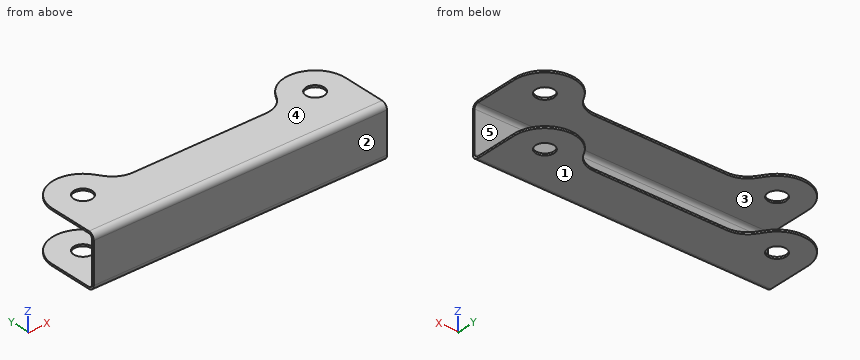
```python
from build123d import *

# Parameters (mm, degrees)
BASE_EXTRUDE_DEPTH         = 13.5
FILLET1_R                  = 12.7
SHELL1_T                   = -1
SKETCH2_R                  = 4.7625
CUT_EXTRUDE1_DEPTH         = 142.468143499
FLATTEN_BENDS1_START       = -24.4
FLATTEN_BENDS1_OUTLINE_W   = 152.4
FLATTEN_BENDS1_OUTLINE_H   = 1
FLATTEN_BENDS1_DEPTH       = 41.4
FLATTEN_BENDS1_START_2     = -25.4
FLATTEN_BENDS1_2_OUTLINE_R = 4.7625
FLATTEN_BENDS1_2_DEPTH     = 1
PROCESS_BENDS1_START       = -54
PROCESS_BENDS1_OUTLINE_W   = 152.4
PROCESS_BENDS1_OUTLINE_H   = 1
PROCESS_BENDS1_DEPTH       = 40.80822
PROCESS_BENDS1_START_2     = 13.19178
PROCESS_BENDS1_2_OUTLINE_W = 152.4
PROCESS_BENDS1_2_OUTLINE_H = 1
PROCESS_BENDS1_2_DEPTH     = 40.80822
PROCESS_BENDS1_START_3     = -13.5
PROCESS_BENDS1_3_OUTLINE_R = 4.7625
PROCESS_BENDS1_3_DEPTH     = 3
PROCESS_BENDS1_START_4     = 10.5
PROCESS_BENDS1_4_OUTLINE_R = 4.7625
PROCESS_BENDS1_4_DEPTH     = 3
PROCESS_BENDS1_START_5     = -15.875
PROCESS_BENDS1_5_DEPTH     = 152.4


with BuildPart() as part:
    # Sketch1 → Base-Extrude (new, symmetric)
    with BuildSketch(Plane.XY):
        with BuildLine():
            Line((-15.875, 0), (-15.875, -25.4))
            Line((-15.875, -25.4), (136.525, -25.4))
            Line((136.525, -25.4), (136.525, 0))
            ThreePointArc((136.525, 0), (123.40666482, 15.633823079), (105.732379645, 5.429569775))
            Line((105.732379645, 5.429569775), (103.756177862, 0))
            Line((103.756177862, 0), (19.379796597, 0))
            Line((19.379796597, 0), (13.004038703, 9.105525927))
            ThreePointArc((13.004038703, 9.105525927), (-4.773704567, 15.140256593), (-15.875, 0))
        make_face()
    extrude(amount=BASE_EXTRUDE_DEPTH, both=True)

    # Fillet1
    # the kernel refuses this fillet: 12.7 mm, written as the material it adds along each edge
    with BuildSketch(Plane(origin=(103.756177862, 0, -13.5), x_dir=(-1, 0, 0), z_dir=(0, 0, 1))) as fillet1_piece_1:
        with BuildLine():
            CenterArc((8.703846213, -12.7), FILLET1_R, 90, 63.612200039)
            Line((-2.672895276, -7.055555556), (-3.810569425, -6.491111111))
            ThreePointArc((-3.810569425, -6.491111111), (-3.169611411, -4.995204193), (-1.193409628, 0.434365582))
            Line((-1.193409628, 0.434365582), (0, 1.27))
            Line((0, 1.27), (8.703846213, 1.27))
            Line((8.703846213, 1.27), (8.703846213, 0))
        make_face()
    extrude(amount=27)
    with BuildSketch(Plane(origin=(19.379796597, 0, 13.5), x_dir=(-0.5735764363510504, 0.8191520442889888, 0), z_dir=(0, 0, -1))) as fillet1_piece_2:
        with BuildLine():
            CenterArc((FILLET1_R * 0.520567050552, FILLET1_R), FILLET1_R, 215, 55)
            Line((-FILLET1_R * 0.298584993737, FILLET1_R * 0.426423563649), (0, 0))
            Line((0, 0), (FILLET1_R * 0.520567050552, 0))
        make_face()
    extrude(amount=27)

    # Shell1
    shell1_openings = [part.faces().sort_by_distance(p)[0] for p in [
        (-15.875, -12.7, 0),
        (136.525, -12.7, 0),
        (124.273424559, 15.45595094, 0),
        (60.521664894, 0, 0),
        (14.29590294, 7.260552593, 0),
        (-4.773704567, 15.140256593, 0),
        (20.126790751, 1.434962419, 0),
        (101.745819363, 1.907075363, 0),
    ]]
    offset(amount=SHELL1_T, openings=shell1_openings, kind=Kind.INTERSECTION)

    # Sketch2 → Cut-Extrude1 (cut, through all)
    with BuildSketch(Plane.XY.offset(13.5)):
        with Locations((120.65, 0)):
            Circle(SKETCH2_R)
        Circle(SKETCH2_R)
    extrude(amount=-CUT_EXTRUDE1_DEPTH, mode=Mode.SUBTRACT)

    # Flatten-Bends1: read off the stored shape, not the designer's step
    # Flatten-Bends1 outline → Flatten-Bends1 (cut)
    with BuildSketch(Plane(origin=(0, 0, 0), x_dir=(1, 0, 0), z_dir=(0, 1, 0)).offset(FLATTEN_BENDS1_START)):
        with Locations((60.325, 13)):
            Rectangle(FLATTEN_BENDS1_OUTLINE_W, FLATTEN_BENDS1_OUTLINE_H)
        with Locations((60.325, -13)):
            Rectangle(FLATTEN_BENDS1_OUTLINE_W, FLATTEN_BENDS1_OUTLINE_H)
    extrude(amount=FLATTEN_BENDS1_DEPTH, mode=Mode.SUBTRACT)

    # Flatten-Bends1 2 outline → Flatten-Bends1 2 (add)
    # profile 1 of 2: a face of its own
    with BuildSketch(Plane(origin=(0, 0, 0), x_dir=(1, 0, 0), z_dir=(0, 1, 0)).offset(FLATTEN_BENDS1_START_2)):
        with BuildLine():
            ThreePointArc((106.429073138, -43.882546373), (124.273424559, -52.282941757), (136.525, -36.826990817))
            Line((136.525, -36.826990817), (136.525, -13.5))
            Line((136.525, -13.5), (-15.875, -13.5))
            Line((-15.875, -13.5), (-15.875, -36.826990817))
            ThreePointArc((-15.875, -36.826990817), (-4.773704567, -51.96724741), (13.004038703, -45.932516744))
            Line((13.004038703, -45.932516744), (15.587767176, -42.242570075))
            ThreePointArc((15.587767176, -42.242570075), (20.126790751, -38.261953236), (25.990998139, -36.826990817))
            Line((25.990998139, -36.826990817), (95.052331649, -36.826990817))
            ThreePointArc((95.052331649, -36.826990817), (101.745819363, -38.73406618), (106.429073138, -43.882546373))
        make_face()
        with Locations((0, -36.826990817)):
            Circle(FLATTEN_BENDS1_2_OUTLINE_R, mode=Mode.SUBTRACT)
        with Locations((120.65, -36.826990817)):
            Circle(FLATTEN_BENDS1_2_OUTLINE_R, mode=Mode.SUBTRACT)
    # profile 2 of 2: a face of its own
    with BuildSketch(Plane(origin=(0, 0, 0), x_dir=(1, 0, 0), z_dir=(0, 1, 0)).offset(FLATTEN_BENDS1_START_2)):
        with BuildLine():
            Line((-15.875, 36.826990817), (-15.875, 13.5))
            Line((-15.875, 13.5), (136.525, 13.5))
            Line((136.525, 13.5), (136.525, 36.826990817))
            ThreePointArc((136.525, 36.826990817), (124.273424559, 52.282941757), (106.429073138, 43.882546373))
            ThreePointArc((106.429073138, 43.882546373), (101.745819363, 38.73406618), (95.052331649, 36.826990817))
            Line((95.052331649, 36.826990817), (25.990998139, 36.826990817))
            ThreePointArc((25.990998139, 36.826990817), (20.126790751, 38.261953236), (15.587767176, 42.242570075))
            Line((15.587767176, 42.242570075), (13.004038703, 45.932516744))
            ThreePointArc((13.004038703, 45.932516744), (-4.773704567, 51.96724741), (-15.875, 36.826990817))
        make_face()
        with Locations((0, 36.826990817)):
            Circle(FLATTEN_BENDS1_2_OUTLINE_R, mode=Mode.SUBTRACT)
        with Locations((120.65, 36.826990817)):
            Circle(FLATTEN_BENDS1_2_OUTLINE_R, mode=Mode.SUBTRACT)
    extrude(amount=FLATTEN_BENDS1_2_DEPTH)

    # Process-Bends1: read off the stored shape, not the designer's step
    # Process-Bends1 outline → Process-Bends1 (cut)
    with BuildSketch(Plane.XY.offset(PROCESS_BENDS1_START)):
        with Locations((60.325, -24.9)):
            Rectangle(PROCESS_BENDS1_OUTLINE_W, PROCESS_BENDS1_OUTLINE_H)
    extrude(amount=PROCESS_BENDS1_DEPTH, mode=Mode.SUBTRACT)

    # Process-Bends1 2 outline → Process-Bends1 2 (cut)
    with BuildSketch(Plane.XY.offset(PROCESS_BENDS1_START_2)):
        with Locations((60.325, -24.9)):
            Rectangle(PROCESS_BENDS1_2_OUTLINE_W, PROCESS_BENDS1_2_OUTLINE_H)
    extrude(amount=PROCESS_BENDS1_2_DEPTH, mode=Mode.SUBTRACT)

    # Process-Bends1 3 outline → Process-Bends1 3 (add)
    with BuildSketch(Plane.XY.offset(PROCESS_BENDS1_START_3)):
        with BuildLine():
            Line((136.525, -24.4), (136.525, 0))
            ThreePointArc((136.525, 0), (124.273424559, 15.45595094), (106.429073138, 7.055555556))
            ThreePointArc((106.429073138, 7.055555556), (101.745819363, 1.907075363), (95.052331649, 0))
            Line((95.052331649, 0), (25.990998139, 0))
            ThreePointArc((25.990998139, 0), (20.126790751, 1.434962419), (15.587767176, 5.415579258))
            Line((15.587767176, 5.415579258), (13.004038703, 9.105525927))
            ThreePointArc((13.004038703, 9.105525927), (-4.773704567, 15.140256593), (-15.875, 0))
            Line((-15.875, 0), (-15.875, -24.4))
            Line((-15.875, -24.4), (136.525, -24.4))
        make_face()
        Circle(PROCESS_BENDS1_3_OUTLINE_R, mode=Mode.SUBTRACT)
        with Locations((120.65, 0)):
            Circle(PROCESS_BENDS1_3_OUTLINE_R, mode=Mode.SUBTRACT)
    extrude(amount=PROCESS_BENDS1_3_DEPTH)

    # Process-Bends1 4 outline → Process-Bends1 4 (add)
    with BuildSketch(Plane.XY.offset(PROCESS_BENDS1_START_4)):
        with BuildLine():
            Line((136.525, -24.4), (136.525, 0))
            ThreePointArc((136.525, 0), (124.273424559, 15.45595094), (106.429073138, 7.055555556))
            ThreePointArc((106.429073138, 7.055555556), (101.745819363, 1.907075363), (95.052331649, 0))
            Line((95.052331649, 0), (25.990998139, 0))
            ThreePointArc((25.990998139, 0), (20.126790751, 1.434962419), (15.587767176, 5.415579258))
            Line((15.587767176, 5.415579258), (13.004038703, 9.105525927))
            ThreePointArc((13.004038703, 9.105525927), (-4.773704567, 15.140256593), (-15.875, 0))
            Line((-15.875, 0), (-15.875, -24.4))
            Line((-15.875, -24.4), (136.525, -24.4))
        make_face()
        Circle(PROCESS_BENDS1_4_OUTLINE_R, mode=Mode.SUBTRACT)
        with Locations((120.65, 0)):
            Circle(PROCESS_BENDS1_4_OUTLINE_R, mode=Mode.SUBTRACT)
    extrude(amount=PROCESS_BENDS1_4_DEPTH)

    # Process-Bends1 5 outline → Process-Bends1 5 (cut)
    with BuildSketch(Plane.YZ.offset(PROCESS_BENDS1_START_5)):
        with BuildLine():
            ThreePointArc((-24.4, -10.5), (-23.814213562, -11.914213562), (-22.4, -12.5))
            Line((-22.4, -12.5), (17, -12.5))
            Line((17, -12.5), (17, -10.5))
            Line((17, -10.5), (-24.4, -10.5))
        make_face()
        with BuildLine():
            Line((0, -15), (0, -13.5))
            Line((0, -13.5), (-22.4, -13.5))
            ThreePointArc((-22.4, -13.5), (-24.521320344, -12.621320344), (-25.4, -10.5))
            Line((-25.4, -10.5), (-25.4, -13.19178))
            Line((-25.4, -13.19178), (-24.4, -13.19178))
            Line((-24.4, -13.19178), (-24.4, -15))
            Line((-24.4, -15), (0, -15))
        make_face()
        with BuildLine():
            ThreePointArc((-22.4, 12.5), (-23.814213562, 11.914213562), (-24.4, 10.5))
            Line((-24.4, 10.5), (17, 10.5))
            Line((17, 10.5), (17, 12.5))
            Line((17, 12.5), (-22.4, 12.5))
        make_face()
        with BuildLine():
            Line((-22.4, 13.5), (0, 13.499999989))
            Line((0, 13.499999989), (0, 15))
            Line((0, 15), (-24.4, 15))
            Line((-24.4, 15), (-24.4, 13.19178))
            Line((-24.4, 13.19178), (-25.4, 13.19178))
            Line((-25.4, 13.19178), (-25.4, 10.5))
            ThreePointArc((-25.4, 10.5), (-24.521320344, 12.621320344), (-22.4, 13.5))
        make_face()
    extrude(amount=PROCESS_BENDS1_5_DEPTH, mode=Mode.SUBTRACT)


solid = part.part
```
Geometry check sheet. Reference: the model listing, model coordinates, mm. Face numbers are marked on the shaded views. A direction names the side the tool comes from. Coordinates: 2 decimals unless noted, no trailing zeros. Order: outer loops, then holes, each group sorted by start corner. A loop starts at its lowest first (then second) coordinate and runs counter-clockwise, first axis right, second up. Notation, with made-up numbers: M -22.5,80.5 L 32.5,80.5 A22 ccw 32.5,107.5 Z; hole C 58.5,35 d4. An arc over 180 degrees is marked long. One line per question, with ' | ' between items. Start each with the question number.
Item 1: Cross-section at C-C on x = 65. Enter the section's corners in (y, z).
Item 2: Cross-section at D-D on z = 1. Enter the section's corners in (x, y) (3 decimals).
Item 3: Gauge pin test, flat ends, axial feed: pin 1 (8 mm diameter, centred on x = 30.5, z = -0.5, fed in from +Y); pin 2 (11 mm diameter, centred on x = 0, y = 0, fed in from -Z); pin 3 (0.5 mm diameter, centred on x = 67.5, z = -13, fed in from +Y); pin 4 (12 mm diameter, centred on y = 7.5, z = -7.5, fed in from +X). Record the tip position at first contact, or that the pin passes through.
Item 4: Cross-section at B-B on y = 3. State how many separate pieces and enclosed holes the cut face has, then the cut area to 3 significant figures.
Item 5: Material ranges on L1, parallel to Z at x = 58, y = -13.5; L2, parallel to Y at x = 120.65, z = 13 (1 decimal); L3, parallel to Y at x = 80.5, z = 5.25, recorded low to high. Write a range as [from, to].
Item 6: Set-up check for the marked faces 4 and 5: record each of +Z, -Z, +X, -X, +Y, -Y from which the full face is reachable in a straight line by a thin tool's end or side.
Item 7: Cross-section at A-A on x = 0. Enter the section's corners in (y, z) (1 decimal).
Item 8: Draft check along Z on the marked faces 1, 2 and 3. Enter one of: pulls with the +Z half, pulls with the -Z half, needs draft (parallel to the pull), parting line crosses it, or undercut.
Findings:
1) outline: M -25.4,-10.5 A3 ccw -22.4,-13.5 L 0,-13.5 L 0,-12.5 L -22.4,-12.5 A2 cw -24.4,-10.5 L -24.4,10.5 A2 cw -22.4,12.5 L 0,12.5 L 0,13.5 L -22.4,13.5 A3 ccw -25.4,10.5 Z
2) outline: M -15.875,-25.4 L 136.525,-25.4 L 136.525,-24.4 L -15.875,-24.4 Z
3) pin 1: stops at y = -24.4 | pin 2: stops at z = -13.5 | pin 3: stops at y = 0 | pin 4: stops at x = 135.96
4) separate pieces: 8 | enclosed holes: 0 | area: 103 mm²
5) L1: z = [-13.5, -12.5], [12.5, 13.5] | L2: y = [-24.1, -4.8], [4.8, 15.9] | L3: y = [-25.4, -24.4]
6) face 4: +Z, +X, -X, +Y, -Y | face 5: +X, -X, +Y
7) outline: M -25.4,-10.5 A3 ccw -22.4,-13.5 L -4.8,-13.5 L -4.8,-12.5 L -22.4,-12.5 A2 cw -24.4,-10.5 L -24.4,10.5 A2 cw -22.4,12.5 L -4.8,12.5 L -4.8,13.5 L -22.4,13.5 A3 ccw -25.4,10.5 Z; M 4.8,-13.5 L 15.9,-13.5 L 15.9,-12.5 L 4.8,-12.5 Z; M 4.8,12.5 L 15.9,12.5 L 15.9,13.5 L 4.8,13.5 Z
8) face 1: pulls with the -Z half | face 2: needs draft | face 3: undercut
